```python
from build123d import *

# Parameters (mm, degrees)
SKETCH_1_W          = 15
SKETCH_1_H          = 10
SKETCH_1_W_2        = 13
SKETCH_1_H_2        = 8
EXTRUDE_1_DEPTH     = 40
SKETCH_2_R          = 2.1
CUT_EXTRUDE_1_DEPTH = 44.011626335
SKETCH_3_R          = 2.1
CUT_EXTRUDE_2_DEPTH = 42.907636536


with BuildPart() as part:
    # ｽｹｯﾁ1 → 押し出し-薄板1 (new body)
    with BuildSketch(Plane(origin=(0, 0, 0), x_dir=(1, 0, 0), z_dir=(0, 1, 0))):
        Rectangle(SKETCH_1_W, SKETCH_1_H)
        Rectangle(SKETCH_1_W_2, SKETCH_1_H_2, mode=Mode.SUBTRACT)
    extrude(amount=EXTRUDE_1_DEPTH)

    # ｽｹｯﾁ2 → ｶｯﾄ - 押し出し1 (cut, through all)
    with BuildSketch(Plane(origin=(7.5, 0, 0), x_dir=(0, 0, -1), z_dir=(1, 0, 0))):
        with Locations((0, 35)):
            Circle(SKETCH_2_R)
        with Locations((0, 5)):
            Circle(SKETCH_2_R)
    extrude(amount=-CUT_EXTRUDE_1_DEPTH, mode=Mode.SUBTRACT)

    # ｽｹｯﾁ3 → ｶｯﾄ - 押し出し2 (cut, through all)
    with BuildSketch(Plane.XY.offset(5)):
        with Locations((0, 30)):
            Circle(SKETCH_3_R)
        with Locations(Location((0, 10, 0), (0, 0, 180))):
            Circle(SKETCH_3_R)
    extrude(amount=-CUT_EXTRUDE_2_DEPTH, mode=Mode.SUBTRACT)


solid = part.part
```
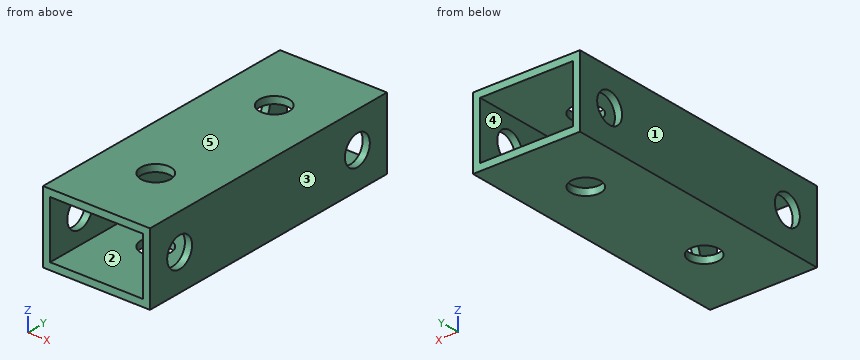
For this review, take the finished solid that the model builds, in its own axes (mm). Face numbers are marked on the shaded views. A direction names the side the tool comes from. Round coordinates to 2 decimals unless told otherwise and drop trailing zeros. Write each loop counter-clockwise with the first axis right and the second up, starting at its lowest first coordinate (ties: lowest second). Pieces come first, ordered by that corner, then holes. Notation, with made-up numbers: (-5.75, 82.25) - (21.25, 82.25) arc R23 ccw to (21.25, 106.25) - close; hole circle Ø8 at (68.5, 84). An arc over 180 degrees is marked (long way). Use CSV: the item, a comma, the result in double quotes.
1) The part is to be moulded in two halves that separate along X. For the marked faces 1, 2 and 3, say which applies: pulls with the +X half, pulls with the -X half, needs draft (parallel to the pull), parting line crosses it, or undercut.
Conclusion:
face 1,"pulls with the -X half"
face 2,"undercut"
face 3,"pulls with the +X half"
2) Add section C-C on y = 10. Write out the cut boundary in (x, z), and give its area (3 significant figures).
Conclusion:
outline,"(-7.5, -5) - (-2.1, -5) - (-2.1, -4) - (-6.5, -4) - (-6.5, 4) - (-2.1, 4) - (-2.1, 5) - (-7.5, 5) - close; (2.1, -5) - (7.5, -5) - (7.5, 5) - (2.1, 5) - (2.1, 4) - (6.5, 4) - (6.5, -4) - (2.1, -4) - close"
area,"37.6 mm^2"
3) Add section D-D on x = 0. Write out the cut boundary in (y, z), and give its area (3 significant figures).
Conclusion:
outline,"(0, -5) - (7.9, -5) - (7.9, -4) - (0, -4) - close; (0, 4) - (7.9, 4) - (7.9, 5) - (0, 5) - close; (12.1, -5) - (27.9, -5) - (27.9, -4) - (12.1, -4) - close; (12.1, 4) - (27.9, 4) - (27.9, 5) - (12.1, 5) - close; (32.1, -5) - (40, -5) - (40, -4) - (32.1, -4) - close; (32.1, 4) - (40, 4) - (40, 5) - (32.1, 5) - close"
area,"63.2 mm^2"
4) Add section B-B on z = 2.5. Write out the cut boundary in (x, y), and give its area (3 significant figures).
Conclusion:
outline,"(-7.5, 0) - (-6.5, 0) - (-6.5, 40) - (-7.5, 40) - close; (6.5, 0) - (7.5, 0) - (7.5, 40) - (6.5, 40) - close"
area,"80.0 mm^2"
5) Add section A-A on x = -3.5. Write out the cut boundary in (y, z), and give its area (3 significant figures).
Conclusion:
outline,"(0, -5) - (40, -5) - (40, -4) - (0, -4) - close; (0, 4) - (40, 4) - (40, 5) - (0, 5) - close"
area,"80.0 mm^2"
6) Wall thickness on line 1 along Y through (x, z) = (0, 4.25); line 2 along X through (y, z) = (12, -1.75); line 3 along Z through (x, y) = (1, 21.5): over which ranges is each line inside the solid? List them lowest first. Write a range as from..to.
Conclusion:
line 1,"y = 0..7.9, 12.1..27.9, 32.1..40"
line 2,"x = -7.5..-6.5, 6.5..7.5"
line 3,"z = -5..-4, 4..5"
7) Clearance check with a flat-ended pin moving along its axis: pin 1 Ø2.5 at (y, z) = (35, 0) entering from -X. State where the tip first meets the part, or that it passes through.
Conclusion:
pin 1,"passes through"
8) For the marked faces 4 and 5, list the 3-axis set-ups (+Z, -Z, +X, -X, +Y, -Y) from which the entire face can be reached by the end or side of a thin tool; tool diameter is ignored.
Conclusion:
face 4,"+Y, -Y"
face 5,"+Z, +X, -X, +Y, -Y"
